Job drawing, mm, ordinate dimensions from the low corner. One solid piece. A direction names the side the tool comes from. Round coordinates to 2 decimals unless told otherwise and drop trailing zeros. Loops run counter-clockwise (first coordinate to the right, second up) from the corner with the lowest first, then second, coordinate; pieces in that order, holes last.
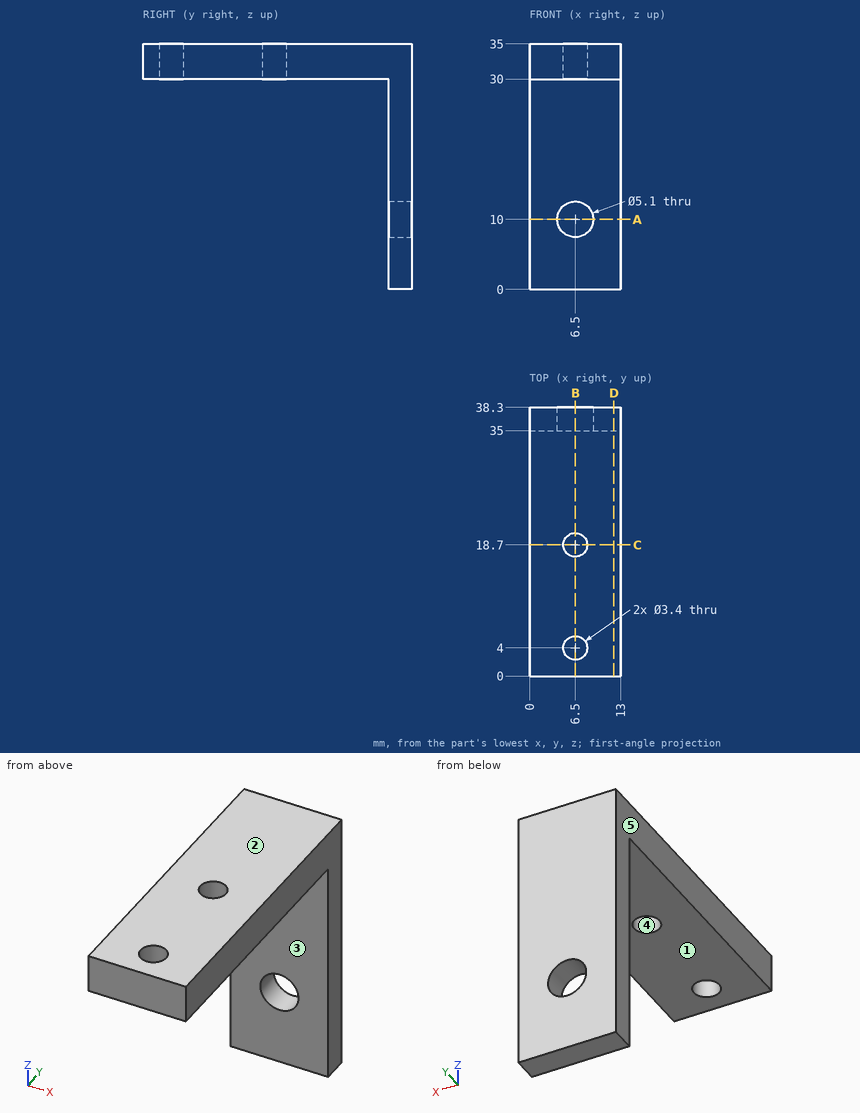
(1) Slice it at A-A on z = 10. List the corners of the cut face in (x, y), plus the area to 3 significant figures.
Responses:
outline: (0, 35) - (3.95, 35) - (3.95, 38.3) - (0, 38.3) - close; (9.05, 35) - (13, 35) - (13, 38.3) - (9.05, 38.3) - close
area: 26.1 mm2
(2) Pin check, flat tips, straight feed: P1, Ø4.5, axis at x = 6.5, y = 4, coming from the -Z side; P2, Ø6, axis at x = 6.5, z = 10, coming from the -Y side; P3, Ø8, axis at y = 30, z = 5, coming from the -X side. Stop position of each tip, or through.
Responses:
P1: stops at z = 30
P2: stops at y = 35
P3: passes through
(3) Probe line 1 (Z direction, x = 6.5, y = 35.75); line 2 (Y direction, x = 6.5, z = 32.4); line 3 (X direction, y = 37.35, z = 10). List the from-to ranges inside material, lowest first.
Responses:
line 1: z = 0 to 7.45, 12.55 to 35
line 2: y = 0 to 2.3, 5.7 to 17, 20.4 to 38.3
line 3: x = 0 to 3.95, 9.05 to 13
(4) Slice it at B-B on x = 6.5. List the corners of the cut face in (y, z).
Responses:
outline: (0, 30) - (2.3, 30) - (2.3, 35) - (0, 35) - close; (5.7, 30) - (17, 30) - (17, 35) - (5.7, 35) - close; (20.4, 30) - (35, 30) - (35, 12.55) - (38.3, 12.55) - (38.3, 35) - (20.4, 35) - close; (35, 0) - (38.3, 0) - (38.3, 7.45) - (35, 7.45) - close
(5) Slice it at D-D on x = 12. List the corners of the cut face in (y, z), plus the area to 4 significant figures.
Responses:
outline: (0, 30) - (35, 30) - (35, 0) - (38.3, 0) - (38.3, 35) - (0, 35) - close
area: 290.5 mm2
(6) Slice it at C-C on y = 18.7. List the corners of the cut face in (x, z).
Responses:
outline: (0, 30) - (4.8, 30) - (4.8, 35) - (0, 35) - close; (8.2, 30) - (13, 30) - (13, 35) - (8.2, 35) - close
(7) Which spindle directions (+Z, -Z, +X, -X, +Y, -Y) get a long thin tool onto all of the face, cutting with end or side? Do the marked faces 1 and 2. Say none if no direction does.
Responses:
face 1: -Z, +X, -X, -Y
face 2: +Z, +X, -X, +Y, -Y
(8) Pull direction X, two halves, no side cores. Call the marked faces 3, 4 and 5: +X half, -X half, draft (parallel to the pull), parting line (faces both ways), or undercut.
Responses:
face 3: draft
face 4: undercut
face 5: -X half
